Source: CAD feature listing. Evaluate the final solid. Frame: model axes, mm. A direction names the side the tool comes from. Round coordinates to 2 decimals unless told otherwise and drop trailing zeros. Write each loop counter-clockwise with the first axis right and the second up, starting at its lowest first coordinate (ties: lowest second). Pieces come first, ordered by that corner, then holes. Notation, with made-up numbers: (-6, 43.25) -> (39, 43.25) arc R17 ccw to (39, 65.25) -> close; hole circle Ø8 at (39, 42). An arc over 180 degrees is marked (long way). Put each result on its own line as item: value.
Solid Edge part; units mm, degrees
sketch "Sketch1" plane through (0, 0, 0) normal (0, 0, 1) x (1, 0, 0)
  line L0 (400, 150) -> (-400, 150)
  line L1 (-400, 150) -> (-400, 0)
  line L2 (-400, 0) -> (400, 0)
  line L3 (400, 0) -> (400, 150)
extrude "Protrusion1" add sketch "Sketch1" along normal blind 20
hole "Hole1" at (-375, 125, 20) direction (0, 0, -1) diameter 6 end through all start chamfer 1 start chamfer angle 45 end chamfer 1 end chamfer angle 45
hole "Hole2" at (-325, 125, 20) direction (0, 0, -1) diameter 6 end through all start chamfer 1 start chamfer angle 45 end chamfer 1 end chamfer angle 45
hole "Hole3" at (-325, 25, 20) direction (0, 0, -1) diameter 6 end through all start chamfer 1 start chamfer angle 45 end chamfer 1 end chamfer angle 45
hole "Hole4" at (-375, 25, 20) direction (0, 0, -1) diameter 6 end through all start chamfer 1 start chamfer angle 45 end chamfer 1 end chamfer angle 45
hole "Hole5" at (325, 125, 20) direction (0, 0, -1) diameter 6 end through all start chamfer 1 start chamfer angle 45 end chamfer 1 end chamfer angle 45
hole "Hole6" at (375, 125, 20) direction (0, 0, -1) diameter 6 end through all start chamfer 1 start chamfer angle 45 end chamfer 1 end chamfer angle 45
hole "Hole7" at (375, 25, 20) direction (0, 0, -1) diameter 6 end through all start chamfer 1 start chamfer angle 45 end chamfer 1 end chamfer angle 45
hole "Hole8" at (325, 25, 20) direction (0, 0, -1) diameter 6 end through all start chamfer 1 start chamfer angle 45 end chamfer 1 end chamfer angle 45
hole "Stufenbohrung_Axiallager" at (0, 50, 20) direction (0, 0, -1) diameter 30 end through all counterbore diameter 47 counterbore depth 10 start chamfer 1 start chamfer angle 45 end chamfer 1 end chamfer angle 45
hole "Hole9" at (-100, 20, 20) direction (0, 0, -1) diameter 6 end through all start chamfer 1 start chamfer angle 45 end chamfer 1 end chamfer angle 45
hole "Hole10" at (100, 20, 20) direction (0, 0, -1) diameter 6 end through all start chamfer 1 start chamfer angle 45 end chamfer 1 end chamfer angle 45
Q1. Material intervals for line 1 (X direction, y = 125, z = 11.5); line 2 (Y direction, x = -325, z = 12.75); line 3 (X direction, y = 20, z = 12), sorted ascending. Write a range as [from, to].
Ans:
line 1: x = [-400, -378], [-372, -328], [-322, 322], [328, 372], [378, 400]
line 2: y = [0, 22], [28, 122], [128, 150]
line 3: x = [-400, -103], [-97, 97], [103, 400]
Q2. Reachability of faces 1 (the cylindrical face through (-15.88, 67.32, 14.44)), 2 (the flat face through (6, 150, 10)) from +Z, -Z, +X, -X, +Y, -Y: full face, straight path, thin tool, end or side. Return the list, or none.
Ans:
face 1: +Z
face 2: +Z, -Z, +X, -X, +Y
Q3. Cut plane A-A on y = 50. Output: boundary loops of the cut face in (x, z).
Ans:
outline: (-400, 0) -> (-16, 0) -> (-15, 1) -> (-15, 10) -> (-23.5, 10) -> (-23.5, 19) -> (-24.5, 20) -> (-400, 20) -> close; (15, 1) -> (16, 0) -> (400, 0) -> (400, 20) -> (24.5, 20) -> (23.5, 19) -> (23.5, 10) -> (15, 10) -> close
Q4. Pin query (flat end, axial travel): pin 1 (5.5 mm diameter, centred on x = 325, y = 125, fed in from +Z); pin 2 (4 mm diameter, centred on x = 9, y = 62, fed in from +Z); pin 3 (7 mm diameter, centred on x = -325, y = 25, fed in from +Z); pin 4 (7 mm diameter, centred on x = 325, y = 25, fed in from -Z). Return the tip coordinate at first contact, or that it passes through.
Ans:
pin 1: passes through
pin 2: stops at z = 10
pin 3: stops at z = 19.5
pin 4: stops at z = 0.5
Q5. Draft query along X for faces 3 (the flat face through (-6, 0, 10)), 4 (the flat face through (-400, 76, 10)), 5 (the flat face through (15.3, 50.3, 10)), 6 (the cylindrical face through (0.66, 64.985, 5.563)). Return one class per face: +X half, -X half, draft (parallel to the pull), parting line (faces both ways), or undercut.
Ans:
face 3: draft
face 4: -X half
face 5: undercut
face 6: undercut
